Verification items for this drawing (mm, ordinates from the low corner). A direction names the side the tool comes from. Round coordinates to 2 decimals unless told otherwise and drop trailing zeros. Loops run counter-clockwise (first coordinate to the right, second up) from the corner with the lowest first, then second, coordinate; pieces in that order, holes last. Notation, with made-up numbers: (77, 80.5) - (135, 80.5) arc R18 cw to (135, 105.5) - close; hole circle Ø9 at (59.5, -5.5). An arc over 180 degrees is marked (long way). Put each result on its own line as item: value. Start each with the question number.
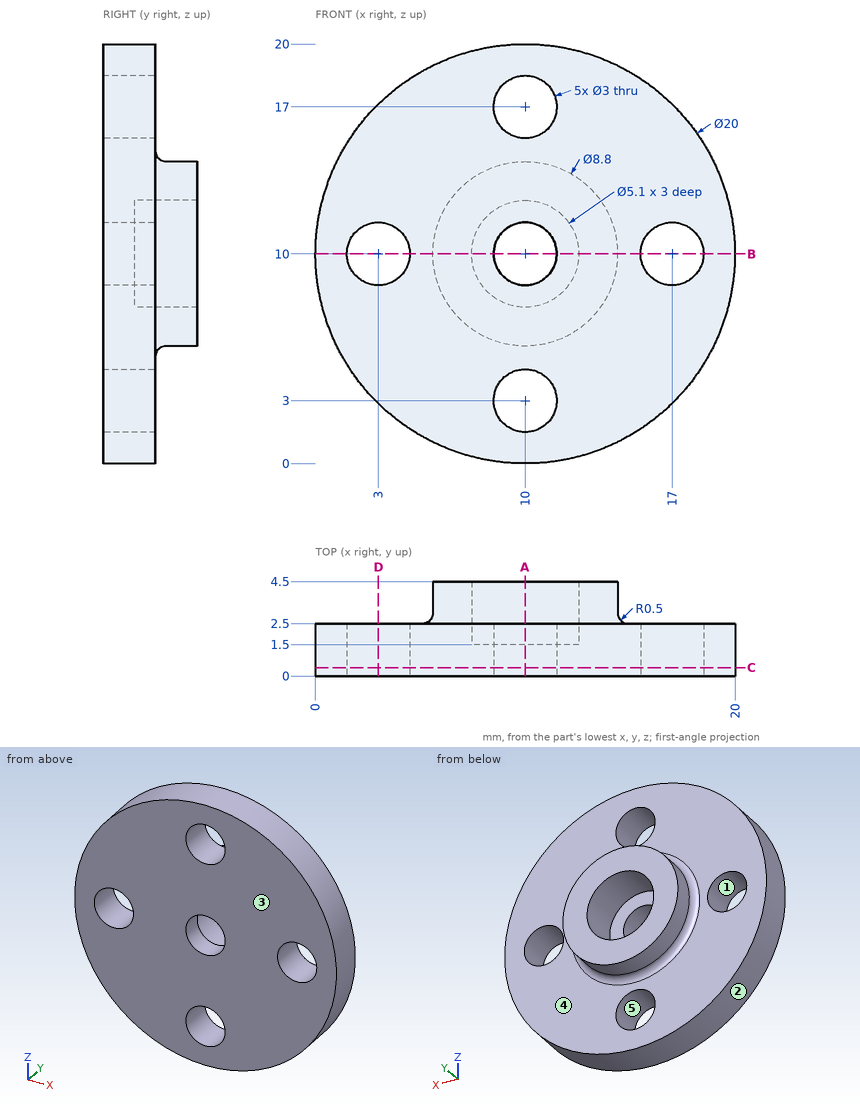
Q1. Cross-section at D-D on x = 3. Enter the section's corners in (y, z), and give its area (3 significant figures).
Q2. Set-up check for the marked faces 4 and 5: record each of +Z, -Z, +X, -X, +Y, -Y from which the full face is reachable in a straight line by a thin tool's end or side.
Q3. Depth check by flat-ended pin: pin 1 Ø1.8 at (x, z) = (3, 10) entering from -Y; pin 2 Ø1.5 at (y, z) = (2, 16.5) entering from +X; pin 3 Ø2 at (x, z) = (17, 2) entering from +Y. Enter the tip coordinate at first touch or a pass-through.
Q4. Material ranges on line 1 (X direction, y = 1.9, z = 11); line 2 (Y direction, x = 3.5, z = 14.25); line 3 (X direction, y = 1.6, z = 16.5), recorded low to high. Write a range as from..to.
Q5. Cross-section at A-A on x = 10. Enter the section's corners in (y, z).
Q6. Draft check along X on the marked faces 1, 2 and 3. Enter one of: +X half, -X half, draft (parallel to the pull), parting line (faces both ways), or undercut.
Q7. Cross-section at B-B on z = 10. Enter the section's corners in (x, y), and give its area (3 significant figures).
Q8. Cross-section at C-C on y = 0.4. Enter the section's corners in (x, z).
Answer list:
1. outline: (0, 2.86) - (2.5, 2.86) - (2.5, 8.5) - (0, 8.5) - close; (0, 11.5) - (2.5, 11.5) - (2.5, 17.14) - (0, 17.14) - close
1. area: 28.2 mm2
2. face 4: +Y
2. face 5: +Y, -Y
3. pin 1: passes through
3. pin 2: stops at x = 18.18
3. pin 3: stops at y = 2.5
4. line 1: x = 0.05..1.88, 4.12..7.65, 12.35..15.88, 18.12..19.95
4. line 2: y = 0..2.5
4. line 3: x = 2.4..8.59, 11.41..17.6
5. outline: (0, 0) - (2.5, 0) - (2.5, 1.5) - (0, 1.5) - close; (0, 4.5) - (2.5, 4.5) - (2.5, 5.1) arc R0.5 cw to (3, 5.6) - (4.5, 5.6) - (4.5, 7.45) - (1.5, 7.45) - (1.5, 8.5) - (0, 8.5) - close; (0, 11.5) - (1.5, 11.5) - (1.5, 12.55) - (4.5, 12.55) - (4.5, 14.4) - (3, 14.4) arc R0.5 cw to (2.5, 14.9) - (2.5, 15.5) - (0, 15.5) - close; (0, 18.5) - (2.5, 18.5) - (2.5, 20) - (0, 20) - close
6. face 1: undercut
6. face 2: parting line
6. face 3: draft
7. outline: (0, 0) - (1.5, 0) - (1.5, 2.5) - (0, 2.5) - close; (4.5, 0) - (8.5, 0) - (8.5, 1.5) - (7.45, 1.5) - (7.45, 4.5) - (5.6, 4.5) - (5.6, 3) arc R0.5 cw to (5.1, 2.5) - (4.5, 2.5) - close; (11.5, 0) - (15.5, 0) - (15.5, 2.5) - (14.9, 2.5) arc R0.5 cw to (14.4, 3) - (14.4, 4.5) - (12.55, 4.5) - (12.55, 1.5) - (11.5, 1.5) - close; (18.5, 0) - (20, 0) - (20, 2.5) - (18.5, 2.5) - close
7. area: 32.9 mm2
8. outline: circle Ø20 at (10, 10); hole circle Ø3 at (3, 10); hole circle Ø3 at (10, 3); hole circle Ø3 at (10, 10); hole circle Ø3 at (10, 17); hole circle Ø3 at (17, 10)
